Input: dimensioned drawing with shaded views. Units: mm. Origin: part minimum x, y, z. Round coordinates to 2 decimals unless told otherwise and drop trailing zeros. Order: outer loops, then holes, each group sorted by start corner. A loop starts at its lowest first (then second) coordinate and runs counter-clockwise, first axis right, second up.
Item 1: Cut plane A-A on x = 31.5. Output: boundary loops of the cut face in (y, z), then the cut area to 3 significant figures.
Item 2: Line query: L1, parallel to Y at x = 30, z = 40; L2, parallel to X at y = 52.5, z = 37.5 (1 decimal); L3, parallel to X at y = 29.5, z = 32.5. Output: solid intervals per line, ascending.
Item 3: Cut plane D-D on y = 46.5. Output: boundary loops of the cut face in (x, z) (3 decimals).
Item 4: First-contact query: pin 1 (1 mm diameter, centred on x = 18.5, z = 46, fed in from +Y); pin 2 (4 mm diameter, centred on x = 18.12, y = 50.57, fed in from +Z); pin 3 (1.5 mm diameter, centred on x = 27, y = 49, fed in from -Z); pin 4 (1 mm diameter, centred on y = 6.5, z = 47, fed in from +X). Flat tips, straight axial feed; report the tip coordinate or a pass-through.
Item 5: Cut plane B-B on y = 5. Output: boundary loops of the cut face in (x, z) (3 decimals), then the cut area to 3 significant figures.
Item 6: Cut plane C-C on z = 27. Give the number of separate pieces and of enclosed holes in the cut face, then the cut area to 3 significant figures.
Item 7: Mould query, pull axis Y, two halves, no side actions, for the marked faces 1, 2 and 3. Classes: released by +Y, released by -Y, zero draft, split by the parting line, or undercut.
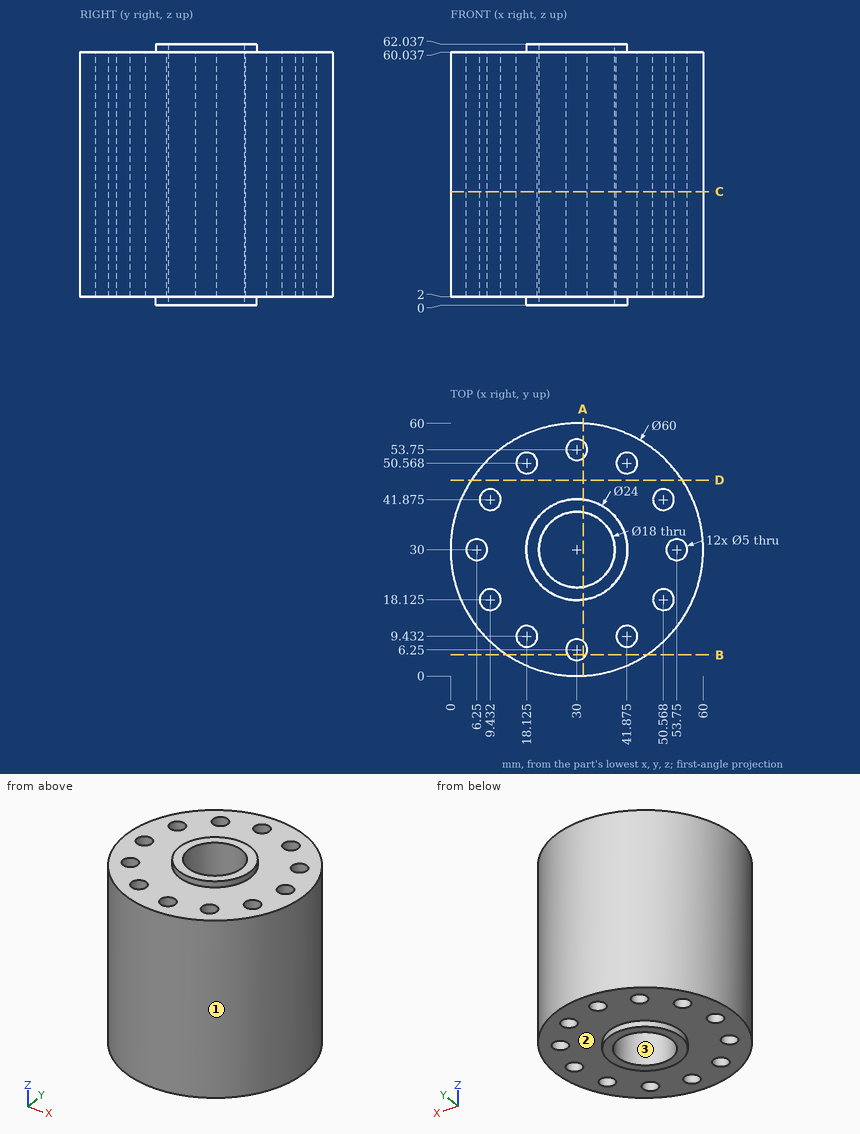
From the geometry:
1. outline: (0.04, 2) - (4.25, 2) - (4.25, 60.04) - (0.04, 60.04) - close; (8.25, 2) - (18.09, 2) - (18.09, 0) - (21.13, 0) - (21.13, 62.04) - (18.09, 62.04) - (18.09, 60.04) - (8.25, 60.04) - close; (38.87, 0) - (41.91, 0) - (41.91, 2) - (51.75, 2) - (51.75, 60.04) - (41.91, 60.04) - (41.91, 62.04) - (38.87, 62.04) - close; (55.75, 2) - (59.96, 2) - (59.96, 60.04) - (55.75, 60.04) - close
1. area: 2,010 mm2
2. L1: y = 0 to 3.75, 8.75 to 21, 39 to 51.25, 56.25 to 60
2. L2: x = 10.2 to 16.5, 19.7 to 27.8, 32.2 to 40.3, 43.5 to 49.8
2. L3: x = 0 to 3.8, 8.7 to 21.01, 38.99 to 51.3, 56.2 to 60
3. outline: (4.945, 2) - (55.055, 2) - (55.055, 60.037) - (4.945, 60.037) - close
4. pin 1: stops at y = 57.91
4. pin 2: passes through
4. pin 3: stops at z = 2
4. pin 4: stops at x = 49.26
5. outline: (13.417, 2) - (27.835, 2) - (27.835, 60.037) - (13.417, 60.037) - close; (32.165, 2) - (46.583, 2) - (46.583, 60.037) - (32.165, 60.037) - close
5. area: 1,670 mm2
6. separate pieces: 1
6. enclosed holes: 13
6. area: 2,340 mm2
7. face 1: split by the parting line
7. face 2: zero draft
7. face 3: undercut
